from build123d import *

# Parameters (mm, degrees)
F1_DEPTH = 25.4
F2_R     = 5.08
F3_DEPTH = 127
F4_R     = 2.54
F5_R     = 2.54
F6_R     = 19.05
F6_R_2   = 5.08
F7_DEPTH = 12.7


with BuildPart() as f1:
    # F0 (on Front) → F1 (new body)
    with BuildSketch(Plane.XZ):
        with BuildLine():
            ThreePointArc((-31.9786, 0), (6.8707, -38.8493), (45.72, 0))
            ThreePointArc((45.72, 0), (0, 45.72), (-45.72, 0))
            Line((-45.72, 0), (-31.9786, 0))
        make_face()
    extrude(amount=F1_DEPTH)

    # F2 (on face) → F3 (cut, symmetric)
    with BuildSketch(Plane.XZ.offset(25.4)):
        Circle(F2_R)
    extrude(amount=F3_DEPTH, both=True, mode=Mode.SUBTRACT)

    # F4
    f4_edges = [f1.edges().sort_by_distance(p)[0] for p in [
        (-45.72, -12.7, 0),
    ]]
    fillet(f4_edges, radius=F4_R)

    # F5
    f5_edges = [f1.edges().sort_by_distance(p)[0] for p in [
        (-31.9786, -12.7, 0),
    ]]
    fillet(f5_edges, radius=F5_R)

    # F6 (on face) → F7 (join)
    with BuildSketch(Plane.XZ.offset(25.4)):
        Circle(F6_R)
        Circle(F6_R_2, mode=Mode.SUBTRACT)
    extrude(amount=F7_DEPTH)


solid = f1.part
Geometry: final body of the model. Coordinates: model frame, mm. A direction names the side the tool comes from. Coordinates: 2 decimals unless noted, no trailing zeros. Loops run counter-clockwise (first coordinate to the right, second up) from the corner with the lowest first, then second, coordinate; pieces in that order, holes last. Notation, with made-up numbers: (-39, 81.25) - (5, 81.25) arc R14 ccw to (5, 100.25) - close; hole circle Ø11 at (-28, 9). An arc over 180 degrees is marked (long way). Put each result on its own line as item: value. Start each with the question number.
Q1. Cut plane A-A, the plane y = -21. Return loops of the section in (x, z), and give its area (3 significant figures).
Q2. Cut plane C-C, the plane z = -9.5. Return loops of the section in (x, y).
Q3. Pull-direction query (X, two-part tool) for faces 4 (the cylindrical face through (-0.661, -18.783, 5.037)), 5 (the cylindrical face through (-44.933, -12.878, 0.777)), 6 (the flat face through (20, -25.4, 4)), 7 (the cylindrical face through (7.226, -12.522, -38.848)); classes: released by +X, released by -X, zero draft, split by the parting line, or undercut.
Q4. Pin query (flat end, axial travel): pin 1 Ø12 at (x, y) = (-21.5, -17) entering from -Z; pin 2 Ø1.5 at (x, z) = (-7, 0.5) entering from +Y; pin 3 Ø10 at (y, z) = (-13, -20) entering from -X; pin 4 Ø10 at (x, y) = (0.5, -30.5) entering from -Z. Return the tip coordinate at first contact, or that it passes through.
Q5. Cut plane B-B, the plane x = 1. Return loops of the section in (y, z), and give its area (3 significant figures).
Q6. Line query: line 1 (Y direction, x = 6.5, z = 25); line 2 (Z direction, x = 0, y = -11); line 3 (X direction, y = -27, z = 2). Output: solid intervals per line, ascending.
Q7. Set-up query: faces 1 (the flat face through (-39, -13, 0)), 2 (the cylindrical face through (-15.12, -31.66, -11.59)), 3 (the cylindrical face through (2.33, -12.52, 45.66)). Return all of +Z, -Z, +X, -X, +Y, -Y with unobstructed straight access to the full face (end or side cutting, diameter ignored); none if empty.
Q8. Cut plane D-D, the plane x = 29. Return loops of the section in (y, z), and give its area (3 significant figures).
Filled sheet:
1. outline: (-45.64, 2.69) arc R2.54 ccw to (-43.11, 0) - (-34.44, 0) arc R2.54 cw to (-31.91, -2.38) arc R38.85 ccw to (45.72, 0) arc R45.72 ccw to start; hole circle Ø10.16 at (0, 0)
1. area: 5,570 mm²
2. outline: (-30.8, -25.4) - (-16.51, -25.4) - (-16.51, -38.1) - (16.51, -38.1) - (16.51, -25.4) - (44.54, -25.4) - (44.54, 0) - (-30.8, 0) - close
3. face 4: undercut
3. face 5: released by -X
3. face 6: zero draft
3. face 7: split by the parting line
4. pin 1: z = -31.76
4. pin 2: y = 0
4. pin 3: x = -28.97
4. pin 4: z = -19.05
5. outline: (-38.1, -19.02) - (-25.4, -19.02) - (-25.4, -38.4) - (0, -38.4) - (0, -4.98) - (-38.1, -4.98) - close; (-38.1, 4.98) - (0, 4.98) - (0, 45.71) - (-25.4, 45.71) - (-25.4, 19.02) - (-38.1, 19.02) - close
5. area: 2,240 mm²
6. line 1: -25.4 to 0
6. line 2: -38.24 to -5.08, 5.08 to 45.72
6. line 3: -18.94 to -4.67, 4.67 to 18.94
7. face 1: -Z, -X, +Y, -Y
7. face 2: -Y
7. face 3: +Z, +Y, -Y
8. outline: (-25.4, -31.93) - (0, -31.93) - (0, 35.35) - (-25.4, 35.35) - close
8. area: 1,710 mm²
